Verification items for the finished model (mm, model axes). Face numbers are marked on the shaded views. A direction names the side the tool comes from. Coordinates: 2 decimals unless noted, no trailing zeros. Write each loop counter-clockwise with the first axis right and the second up, starting at its lowest first coordinate (ties: lowest second). Pieces come first, ordered by that corner, then holes. Notation, with made-up numbers: (43.25, -39) - (93.25, -39) arc R9 cw to (93.25, -29) - close; hole circle Ø2 at (41, -5.5). An arc over 180 degrees is marked (long way). Answer as CSV lines item,"result". Start each with the question number.
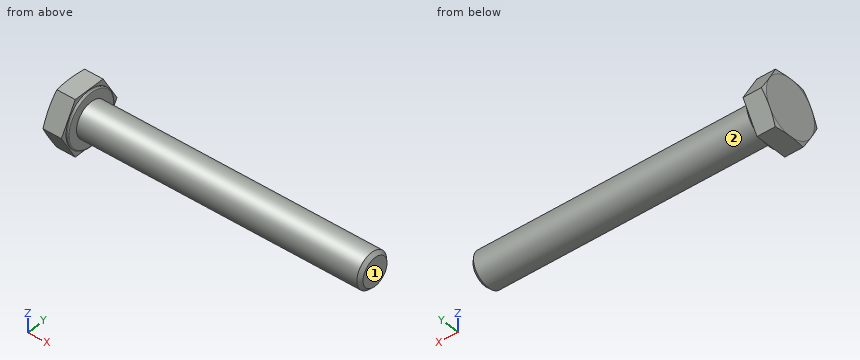
```python
from build123d import *

# Parameters (mm, degrees)
SKETCH_2_W          = 52
SKETCH_2_H          = 52
CUT_EXTRUDE_1_DEPTH = 4.5


with BuildPart() as part:
    # Sketch 1 → Revolve 1 (revolve)
    with BuildSketch(Plane.XY, mode=Mode.PRIVATE) as revolve_1_sk:
        with BuildLine():
            Line((0, 0), (0, 6.5))
            Line((0, 6.5), (0.34833395, 7.8))
            Line((0.34833395, 7.8), (4.5, 7.8))
            Line((4.5, 7.8), (4.5, 6.25))
            Line((4.5, 6.25), (4.75, 6.25))
            ThreePointArc((4.75, 6.25), (4.926776695, 6.176776695), (5, 6))
            Line((5, 6), (5, 4))
            Line((5, 4), (69.533, 4))
            Line((69.533, 4), (70.3, 3.233))
            Line((70.3, 3.233), (70.3, 0))
            Line((70.3, 0), (0, 0))
        make_face()
    revolve(revolve_1_sk.sketch.rotate(Axis((70.3, 0, 0), (-1, 0, 0)), 270), axis=Axis((70.3, 0, 0), (-1, 0, 0)))

    # Sketch 2 → Cut-Extrude 1 (cut)
    with BuildSketch(Plane(origin=(0, 0, 0), x_dir=(0, 0, -1), z_dir=(1, 0, 0))):
        Rectangle(SKETCH_2_W, SKETCH_2_H)
        Polygon((-6.5, 3.75277675), (-6.5, -3.75277675), (0, -7.505553499), (6.5, -3.75277675), (6.5, 3.75277675), (0, 7.505553499), align=None, mode=Mode.SUBTRACT)
    extrude(amount=CUT_EXTRUDE_1_DEPTH, mode=Mode.SUBTRACT)


solid = part.part
```
1. Depth check by flat-ended pin: P1, Ø1.5, axis at x = 30.5, z = 3, coming from the +Y side; P2, Ø3, axis at y = -3, z = 4, coming from the +X side; P3, Ø1.5, axis at y = -5, z = -1, coming from the +X side. Enter the tip coordinate at first touch or a pass-through.
2. Cross-section at A-A (x = 25). Record the cut outline in (y, z), and give its area (3 significant figures).
3. Scan lines: line 1 along Z through (x, y) = (24, 0.25); line 2 along X through (y, z) = (2.75, 5.25); line 3 along X through (y, z) = (5, -4). Record each from-to range of solid material in increasing order. Write a range as from..to.
4. Access from +Z, -Z, +X, -X, +Y, -Y to the whole of each face (thin tool, end or side, straight path). Record for the marked faces 1 and 2.
Completed:
1,P1,"stops at y = 3.31"
1,P2,"stops at x = 70.03"
1,P3,"stops at x = 5"
2,outline,"circle Ø8 at (0, 0)"
2,area,"50.3 mm2"
3,line 1,"z = -3.99..3.99"
3,line 2,"x = 0..5"
3,line 3,"x = 0..4.5"
4,face 1,"+Z, -Z, +X, +Y, -Y"
4,face 2,"+X"
